Source: CAD feature listing. Evaluate the final solid. Frame: model axes, mm. A direction names the side the tool comes from. Round coordinates to 2 decimals unless told otherwise and drop trailing zeros. Write each loop counter-clockwise with the first axis right and the second up, starting at its lowest first coordinate (ties: lowest second). Pieces come first, ordered by that corner, then holes. Notation, with made-up numbers: (26.25, 85.25) -> (60.25, 85.25) arc R22 ccw to (60.25, 120.25) -> close; hole circle Ø4 at (-23, -36). An arc over 180 degrees is marked (long way). Return JSON: item names as keys, results as strings. Group by question number.
from build123d import *

# Parameters (mm, degrees)
F1_DEPTH = 1


with BuildPart() as f1:
    # F0 (on Front) → F1 (new body)
    with BuildSketch(Plane.XZ):
        with BuildLine():
            Line((1, -0.5773502692), (0, 0))
            Line((0, 0), (1, 0.5773502692))
            Line((1, 0.5773502692), (-21.1506350946, 13.3660254038))
            ThreePointArc((-21.1506350946, 13.3660254038), (-44.3012701892, 0), (-21.1506350946, -13.3660254038))
            Line((-21.1506350946, -13.3660254038), (1, -0.5773502692))
        make_face()
        with BuildLine():
            Line((0, 0), (-21.6506350946, -12.5))
            ThreePointArc((-21.6506350946, -12.5), (-43.3012701892, 0), (-21.6506350946, 12.5))
            Line((-21.6506350946, 12.5), (0, 0))
        make_face(mode=Mode.SUBTRACT)
        Polygon((1, 0.5773502692), (0, 0), (1, -0.5773502692), (2, 0), align=None)
        with BuildLine():
            Line((21.6506350946, 12.5), (1, 0.5773502692))
            Line((1, 0.5773502692), (2, 0))
            Line((2, 0), (1, -0.5773502692))
            Line((1, -0.5773502692), (21.6506350946, -12.5))
            ThreePointArc((21.6506350946, -12.5), (43.3012701892, 0), (21.6506350946, 12.5))
        make_face()
        with BuildLine():
            Line((22.1506350946, -11.6339745962), (2, 0))
            Line((2, 0), (22.1506350946, 11.6339745962))
            ThreePointArc((22.1506350946, 11.6339745962), (42.3012701892, 0), (22.1506350946, -11.6339745962))
        make_face(mode=Mode.SUBTRACT)
    extrude(amount=F1_DEPTH)


solid = f1.part
Item 1: Cut plane D-D on z = -10.5. Output: boundary loops of the cut face in (x, y), and give its area (3 significant figures).
Item 2: Set-up query: faces 4 (the flat face through (-10.98, -0.49, 6.34)), 5 (the flat face through (-10.23, -0.49, -7.06)), 6 (the flat face through (11.47, -0.49, 6.62)). Return all of +Z, -Z, +X, -X, +Y, -Y with unobstructed straight access to the full face (end or side cutting, diameter ignored); none if empty.
Item 3: Cut plane B-B on y = -0.6. Output: boundary loops of the cut face in (x, z), and give its area (3 significant figures).
Item 4: Cut plane C-C on x = 37.5. Output: boundary loops of the cut face in (y, z), and give its area (3 significant figures).
Item 5: Cut plane A-A on z = 8. Output: boundary loops of the cut face in (x, y), and give its area (3 significant figures).
Item 6: Material intervals for probe 1 along X at (y, z) = (-0.05, 12); probe 2 along X at (y, z) = (-0.3, -11.5); probe 3 along Z at (x, y) = (37.5, -0.2), sorted ascending.
Item 7: Pull-direction query (Z, two-part tool) for faces 1 (the flat face through (-9.92, -0.49, 6.88)), 2 (the flat face through (-10.67, -0.49, -6.16)), 3 (the cylindrical face through (-44.295, -0.493, 0.452)); classes: +Z half, -Z half, draft (parallel to the pull), parting line (faces both ways), or undercut.
Here are the results:
{
 "1": {"outline": "(-40.18, -1) -> (-38.77, -1) -> (-38.77, 0) -> (-40.18, 0) -> close; (-18.19, -1) -> (-16.19, -1) -> (-16.19, 0) -> (-18.19, 0) -> close; (18.19, -1) -> (20.19, -1) -> (20.19, 0) -> (18.19, 0) -> close; (37.25, -1) -> (38.77, -1) -> (38.77, 0) -> (37.25, 0) -> close", "area": "6.93 mm^2"},
 "2": {"face 4": "+Y, -Y", "face 5": "-Z, +Y, -Y", "face 6": "+Z, +Y, -Y"},
 "3": {"outline": "(-21.15, -13.37) -> (1, -0.58) -> (21.65, -12.5) arc R14.43 ccw (long way) to (21.65, 12.5) -> (1, 0.58) -> (-21.15, 13.37) arc R15.43 ccw (long way) to start; hole (-21.65, -12.5) -> (0, 0) -> (-21.65, 12.5) arc R14.43 ccw (long way) to start; hole (2, 0) -> (22.15, -11.63) arc R13.43 ccw (long way) to (22.15, 11.63) -> close", "area": "220 mm^2"},
 "4": {"outline": "(-1, -11.57) -> (0, -11.57) -> (0, -10.29) -> (-1, -10.29) -> close; (-1, 10.29) -> (0, 10.29) -> (0, 11.57) -> (-1, 11.57) -> close", "area": "2.55 mm^2"},
 "5": {"outline": "(-42.07, -1) -> (-40.88, -1) -> (-40.88, 0) -> (-42.07, 0) -> close; (-13.86, -1) -> (-11.86, -1) -> (-11.86, 0) -> (-13.86, 0) -> close; (13.86, -1) -> (15.86, -1) -> (15.86, 0) -> (13.86, 0) -> close; (39.66, -1) -> (40.88, -1) -> (40.88, 0) -> (39.66, 0) -> close", "area": "6.41 mm^2"},
 "6": {"probe 1": "x = -38.57 to -36.89, -20.78 to -18.78, 20.78 to 22.83, 34.91 to 36.89", "probe 2": "x = -39.16 to -37.59, -19.92 to -17.92, 19.92 to 21.92, 35.81 to 37.59", "probe 3": "z = -11.57 to -10.29, 10.29 to 11.57"},
 "7": {"face 1": "+Z half", "face 2": "undercut", "face 3": "parting line"}
}
